Verification items for the finished model (mm, model axes). Face numbers are marked on the shaded views. A direction names the side the tool comes from. Coordinates: 2 decimals unless noted, no trailing zeros. Order: outer loops, then holes, each group sorted by start corner. A loop starts at its lowest first (then second) coordinate and runs counter-clockwise, first axis right, second up.
Q1. Depth check by flat-ended pin: P1, Ø3, axis at x = -2, y = -19, coming from the -Z side; P2, Ø0.8, axis at x = 0, z = 1.5, coming from the +Y side; P3, Ø2, axis at y = -25.5, z = -0.5, coming from the -X side. Enter the tip coordinate at first touch or a pass-through.
Q2. Cross-section at A-A, the plane z = 0. Record the boundary of the cut face in (x, y).
Q3. Cross-section at B-B, the plane x = 0. Record the boundary of the cut face in (y, z) (3 decimals).
Q4. Thickness scan on line 1 (Z direction, x = -1, y = -19); line 2 (Y direction, x = 3.5, z = -0.5); line 3 (Y direction, x = 3.5, z = 1). Record the ranges inside material, lowest first.
Q5. Set-up check for the marked faces 1 and 2: record each of +Z, -Z, +X, -X, +Y, -Y from which the full face is reachable in a straight line by a thin tool's end or side.
Q6. Cross-section at C-C, the plane y = -8.5. Record the boundary of the cut face in (x, z).
from build123d import *

# Parameters (mm, degrees)
SKETCH7_W           = 1
SKETCH7_H           = 8.308245604
CUT_EXTRUDE3_DEPTH  = 0.5
SKETCH8_R           = 1.5
BOSS_EXTRUDE3_DEPTH = 33.2


with BuildPart() as part:
    # Sketch6 → Revolve1 (revolve)
    with BuildSketch(Plane.XY, mode=Mode.PRIVATE) as revolve1_sk:
        Polygon((0, 0), (4, 0), (1.5, -2), (0, -2), align=None)
    revolve(revolve1_sk.sketch.rotate(Axis((0, 0, 0), (0, 1, 0)), 90), axis=Axis((0, 0, 0), (0, 1, 0)))

    # Sketch7 → Cut-Extrude3 (cut)
    with BuildSketch(Plane(origin=(0, 0, 0), x_dir=(1, 0, 0), z_dir=(0, 1, 0))):
        Rectangle(SKETCH7_W, SKETCH7_H)
    extrude(amount=-CUT_EXTRUDE3_DEPTH, mode=Mode.SUBTRACT)

    # Sketch8 → Boss-Extrude3 (add)
    with BuildSketch(Plane.XZ.offset(2)):
        with Locations(Location((0, 0, 0), (0, 0, 90))):
            Circle(SKETCH8_R)
    extrude(amount=BOSS_EXTRUDE3_DEPTH)


solid = part.part
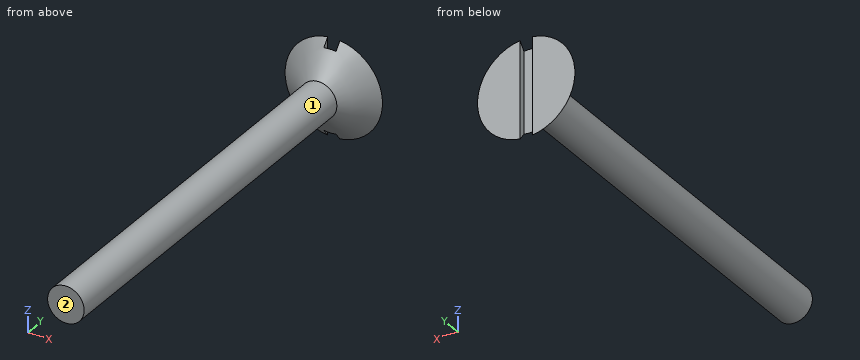
Check values:
1. P1: stops at z = -1.41
1. P2: stops at y = -0.5
1. P3: stops at x = -1.5
2. outline: (-4, 0) - (-1.5, -2) - (-1.5, -35.2) - (1.5, -35.2) - (1.5, -2) - (4, 0) - (0.5, 0) - (0.5, -0.5) - (-0.5, -0.5) - (-0.5, 0) - close
3. outline: (-35.2, -1.5) - (-2, -1.5) - (-0.5, -3.375) - (-0.5, 3.375) - (-2, 1.5) - (-35.2, 1.5) - close
4. line 1: z = -1.12 to 1.12
4. line 2: y = -0.37 to 0
4. line 3: y = -0.29 to 0
5. face 1: -Y
5. face 2: +Z, -Z, +X, -X, -Y
6. outline: circle Ø3 at (0, 0)
